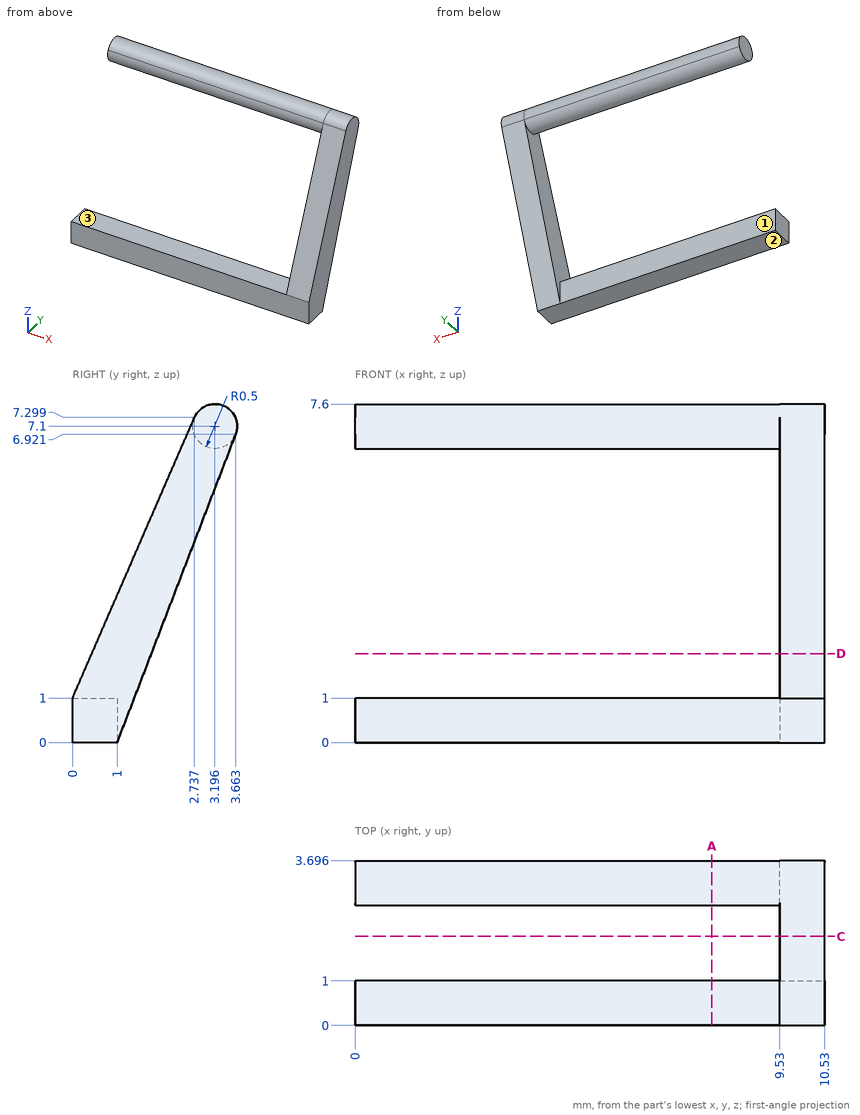
Can you work these out from the drawing? Everything is in mm from the part's minimum corner. A direction names the side the tool comes from. Give positions to 0.01 mm unless a question says otherwise; leave off trailing zeros. Order: outer loops, then holes, each group sorted by start corner. A loop starts at its lowest first (then second) coordinate and runs counter-clockwise, first axis right, second up. Notation, with made-up numbers: M 9.25,-30.75 L 63.25,-30.75 A33 ccw 63.25,7.25 Z; hole C -3.75,58 d7. An arc over 180 degrees is marked long. Write item = value, one per line. Start each with the question number.
Q1. Will these pins go through, and if not, where does the flat tip stop? pin 1 Ø1.1 at (y, z) = (2, 4) entering from -X; pin 2 Ø1.1 at (x, z) = (3, 0.5) entering from +Y.
Q2. For the marked faces 1, 2 and 3, which set-ups out of +Z, -Z, +X, -X, +Y, -Y let a thin tool reach every point of the face, with its end or its side?
Q3. Suppose I cut it at D-D (z = 2). Write out the boundary of the cut face in (x, y) (1 decimal).
Q4. I need wall thicknesses on probe 1 along X at (y, z) = (0.85, 2.25); probe 2 along Z at (x, y) = (4.25, 0.95); probe 3 along Z at (x, y) = (2, 3.5) (1 decimal). Which ranges of each line are inside material? Lowest first, please. Write a range as [from, to].
Q5. Suppose I cut it at C-C (y = 2). Write out the boundary of the cut face in (x, z).
Q6. Suppose I cut it at A-A (x = 8). Write out the boundary of the cut face in (y, z) (1 decimal).
Check result:
q1.pin_1 = 9.53
q1.pin_2 = 1
q2.face_1 = +Z, -Z, -X, +Y
q2.face_2 = -Z, +X, -X, +Y, -Y
q2.face_3 = +Z, -X, +Y, -Y
q3.outline = M 9.5,0.4 L 10.5,0.4 L 10.5,1.8 L 9.5,1.8 Z
q4.probe_1 = [9.53, 10.53]
q4.probe_2 = [0, 1]
q4.probe_3 = [6.7, 7.5]
q5.outline = M 9.53,2.6 L 10.53,2.6 L 10.53,5.6 L 9.53,5.6 Z
q6.outline = M 0,0 L 1,0 L 1,1 L 0,1 Z; M 2.7,7.3 A0.5 ccw long 3.7,6.9 A0.5 ccw Z
